Geometry check sheet. Reference: the model listing, model coordinates, mm. Give positions to 0.01 mm unless a question says otherwise; leave off trailing zeros. Loops run counter-clockwise (first coordinate to the right, second up) from the corner with the lowest first, then second, coordinate; pieces in that order, holes last. Notation, with made-up numbers: (37, 11) -> (69, 11) arc R23 cw to (69, 39) -> close; hole circle Ø7 at (41, 13.5). An arc over 180 degrees is marked (long way). Answer in a Markdown table with one row per item. Add a question column.
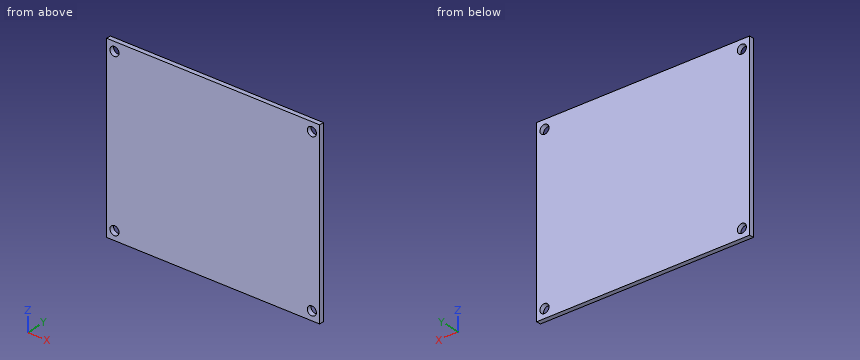
```python
from build123d import *

# Parameters (mm, degrees)
SKETCH1_W                     = 94
SKETCH1_H                     = 79
BASE_FLANGE1_DEPTH            = 2
F_4_0MM_START                 = -2
F_4_0MM_DOWEL_HOLE1_OUTLINE_R = 2
F_4_0MM_DOWEL_HOLE1_DEPTH     = 2


# Read off the part's stored shape, not the designer's step: Ø4.0mm Dowel Hole1
# Sheet-metal steps are written as plain solids
with BuildPart() as part:
    # Sketch1 → Base-Flange1 (new body)
    with BuildSketch(Plane(origin=(0, 0, 0), x_dir=(1, 0, 0), z_dir=(0, 1, 0))):
        Rectangle(SKETCH1_W, SKETCH1_H)
    extrude(amount=-BASE_FLANGE1_DEPTH)

    # Ø4.0mm Dowel Hole1 outline → Ø4.0mm Dowel Hole1 (cut)
    with BuildSketch(Plane(origin=(0, 0, 0), x_dir=(1, 0, 0), z_dir=(0, 1, 0)).offset(F_4_0MM_START)):
        with Locations((43.55, 35.55)):
            Circle(F_4_0MM_DOWEL_HOLE1_OUTLINE_R)
        with Locations((-43.55, -35.55)):
            Circle(F_4_0MM_DOWEL_HOLE1_OUTLINE_R)
        with Locations((-43.55, 35.55)):
            Circle(F_4_0MM_DOWEL_HOLE1_OUTLINE_R)
        with Locations((43.55, -35.55)):
            Circle(F_4_0MM_DOWEL_HOLE1_OUTLINE_R)
    extrude(amount=F_4_0MM_DOWEL_HOLE1_DEPTH, mode=Mode.SUBTRACT)


solid = part.part
```
1. Gauge pin test, flat ends, axial feed: pin 1 Ø2 at (x, z) = (34.5, -27.5) entering from +Y; pin 2 Ø3.5 at (x, z) = (43.55, -35.55) entering from +Y. Record the tip position at first contact, or that the pin passes through.
2. Sectioned sample at A-A (z = 35.55). Enter the section's corners in (x, y), plus the area to 3 significant figures.
3. Sectioned sample at B-B (x = -43.55). Enter the section's corners in (y, z), plus the area to 3 significant figures.
4. Material ranges on L1, parallel to X at y = -1.45, z = -35.55; L2, parallel to Z at x = 43.55, y = -0.8, recorded low to high. Write a range as from..to.
Response:
| question | item | result |
|---|---|---|
| 1 | pin 1 | stops at y = 0 |
| 1 | pin 2 | passes through |
| 2 | outline | (-47, -2) -> (-45.55, -2) -> (-45.55, 0) -> (-47, 0) -> close; (-41.55, -2) -> (41.55, -2) -> (41.55, 0) -> (-41.55, 0) -> close; (45.55, -2) -> (47, -2) -> (47, 0) -> (45.55, 0) -> close |
| 2 | area | 172 mm2 |
| 3 | outline | (-2, -39.5) -> (0, -39.5) -> (0, -37.55) -> (-2, -37.55) -> close; (-2, -33.55) -> (0, -33.55) -> (0, 33.55) -> (-2, 33.55) -> close; (-2, 37.55) -> (0, 37.55) -> (0, 39.5) -> (-2, 39.5) -> close |
| 3 | area | 142 mm2 |
| 4 | L1 | x = -47..-45.55, -41.55..41.55, 45.55..47 |
| 4 | L2 | z = -39.5..-37.55, -33.55..33.55, 37.55..39.5 |
